from build123d import *

# Parameters (mm, degrees)
SKETCH1_R           = 3
SKETCH1_R_2         = 1.5
BOSS_EXTRUDE1_DEPTH = 10
SKETCH2_R           = 1.5
BOSS_EXTRUDE2_DEPTH = 10


with BuildPart() as part:
    # Sketch1 → Boss-Extrude1 (new body)
    with BuildSketch(Plane(origin=(0, 0, 0), x_dir=(1, 0, 0), z_dir=(0, 1, 0))):
        with BuildLine():
            Line((0, -6), (-124, -6))
            ThreePointArc((-124, -6), (-130, 0), (-124, 6))
            Line((-124, 6), (0, 6))
            ThreePointArc((0, 6), (6, 0), (0, -6))
        make_face()
        Circle(SKETCH1_R, mode=Mode.SUBTRACT)
        with Locations((-124, 0)):
            Circle(SKETCH1_R_2, mode=Mode.SUBTRACT)
    extrude(amount=BOSS_EXTRUDE1_DEPTH)

    # Sketch2 → Boss-Extrude2 (add)
    with BuildSketch(Plane(origin=(0, 10, 0), x_dir=(1, 0, 0), z_dir=(0, 1, 0))):
        with BuildLine():
            Line((-119, -24), (-124, -24))
            ThreePointArc((-124, -24), (-130, -30), (-124, -36))
            Line((-124, -36), (-114, -36))
            Line((-114, -36), (-84, -6))
            Line((-84, -6), (-101, -6))
            Line((-101, -6), (-119, -24))
        make_face()
        with Locations((-124, -30)):
            Circle(SKETCH2_R, mode=Mode.SUBTRACT)
    extrude(amount=-BOSS_EXTRUDE2_DEPTH)


solid = part.part
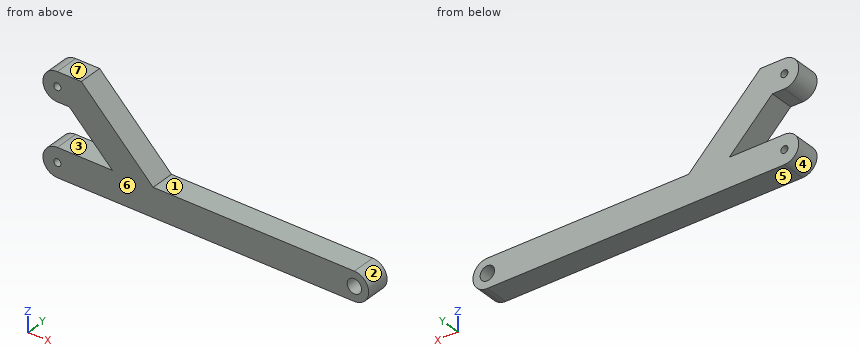
Input: part model. Units: mm. Frame: model coordinates. Face numbers are marked on the shaded views. A direction names the side the tool comes from. Round coordinates to 2 decimals unless told otherwise and drop trailing zeros. Write each loop counter-clockwise with the first axis right and the second up, starting at its lowest first coordinate (ties: lowest second). Pieces come first, ordered by that corner, then holes.
1) Cut plane B-B (z = 0). Return the cut outline in (x, y).
2) Ray query, L1, parallel to X at y = 2.5, z = 0; L2, parallel to Z at x = -124, y = 4.5; L3, parallel to Z at x = 0, y = 6.5. Return the intervals inside material, ascending.
3) Cut plane C-C (y = 8.75). Return the cut outline in (x, z).
4) Cut plane A-A (z = 30). Return the cut outline in (x, y).
5) Reachability of the marked faces 1, 2 and 3 from +Z, -Z, +X, -X, +Y, -Y: full face, straight path, thin tool, end or side. Return the list, or none.
6) Contact query for flat-ended pins moving along their axis: P1, Ø3, axis at y = 9, z = 19, coming from the -X side; P2, Ø1.5, axis at y = 8, z = 20.5, coming from the +X side. Output: stop coordinate, or through.
7) Draft query along Z for the marked faces 4, 5, 6 and 7. Return one class per face: pulls with the +Z half, pulls with the -Z half, needs draft (parallel to the pull), parting line crosses it, or undercut.
8) Cut plane D-D (x = -45). Return the cut outline in (y, z).
Geometry says:
1. outline: (-130, 0) - (-125.5, 0) - (-125.5, 10) - (-130, 10) - close; (-122.5, 0) - (-3, 0) - (-3, 10) - (-122.5, 10) - close; (3, 0) - (6, 0) - (6, 10) - (3, 10) - close
2. L1: x = -130 to -125.5, -122.5 to -3, 3 to 6
2. L2: z = -6 to -1.5, 1.5 to 6, 24 to 28.5, 31.5 to 36
2. L3: z = -6 to -3, 3 to 6
3. outline: (-124, -6) - (0, -6) arc R6 ccw to (0, 6) - (-84, 6) - (-114, 36) - (-124, 36) arc R6 ccw to (-124, 24) - (-119, 24) - (-101, 6) - (-124, 6) arc R6 ccw to start; hole circle Ø3 at (-124, 0); hole circle Ø3 at (-124, 30); hole circle Ø6 at (0, 0)
4. outline: (-130, 0) - (-125.5, 0) - (-125.5, 10) - (-130, 10) - close; (-122.5, 0) - (-108, 0) - (-108, 10) - (-122.5, 10) - close
5. face 1: +Z, +X, +Y, -Y
5. face 2: +X, +Y, -Y
5. face 3: -X, +Y, -Y
6. P1: stops at x = -115.5
6. P2: stops at x = -97.75
7. face 4: undercut
7. face 5: pulls with the -Z half
7. face 6: needs draft
7. face 7: pulls with the +Z half
8. outline: (0, -6) - (10, -6) - (10, 6) - (0, 6) - close
